from build123d import *

# Parameters (mm, degrees)
BOSS_EXTRUDE1_DEPTH = 4
SKETCH3_R           = 2
SKETCH3_R_2         = 2.25
CUT_EXTRUDE1_DEPTH  = 4


with BuildPart() as part:
    # Sketch2 → Boss-Extrude1 (new body)
    with BuildSketch(Plane.XY):
        with BuildLine():
            Line((94.375415976, -52.704406223), (94.375415976, -56.704406223))
            ThreePointArc((94.375415976, -56.704406223), (94.228969367, -57.057959614), (93.875415976, -57.204406223))
            Line((93.875415976, -57.204406223), (86.375415976, -57.204406223))
            ThreePointArc((86.375415976, -57.204406223), (86.021862586, -57.350852833), (85.875415976, -57.704406223))
            Line((85.875415976, -57.704406223), (85.875415976, -59.204406223))
            ThreePointArc((85.875415976, -59.204406223), (86.021862586, -59.557959614), (86.375415976, -59.704406223))
            Line((86.375415976, -59.704406223), (96.375415976, -59.704406223))
            ThreePointArc((96.375415976, -59.704406223), (96.728969367, -59.557959614), (96.875415976, -59.204406223))
            Line((96.875415976, -59.204406223), (96.875415976, -52.704406223))
            ThreePointArc((96.875415976, -52.704406223), (97.021862586, -52.350852833), (97.375415976, -52.204406223))
            Line((97.375415976, -52.204406223), (100.375415976, -52.204406223))
            ThreePointArc((100.375415976, -52.204406223), (106.756191002, -49.976139831), (110.36270914, -44.260154531))
            Line((110.36270914, -44.260154531), (122.04253828, 6.330743606))
            ThreePointArc((122.04253828, 6.330743606), (125.561092562, 11.907314631), (131.786238928, 14.081233063))
            Line((131.786238928, 14.081233063), (170.7844924, 14.081233063))
            ThreePointArc((170.7844924, 14.081233063), (180.903868338, 9.889650306), (185.095451094, -0.229725632))
            Line((185.095451094, -0.229725632), (185.095451094, -11.229725632))
            ThreePointArc((185.095451094, -11.229725632), (184.144121557, -18.570812299), (181.352982104, -25.42691337))
            ThreePointArc((181.352982104, -25.42691337), (169.65700257, -52.25234878), (163.771733482, -80.918766937))
            ThreePointArc((163.771733482, -80.918766937), (169.65700257, -109.585185095), (181.352982104, -136.410620505))
            ThreePointArc((181.352982104, -136.410620505), (184.144121557, -143.266721576), (185.095451094, -150.607808243))
            Line((185.095451094, -150.607808243), (185.095451094, -161.607808243))
            ThreePointArc((185.095451094, -161.607808243), (180.903868338, -171.727184181), (170.7844924, -175.918766937))
            Line((170.7844924, -175.918766937), (131.786238928, -175.918766937))
            ThreePointArc((131.786238928, -175.918766937), (125.561092562, -173.744848506), (122.04253828, -168.168277481))
            Line((122.04253828, -168.168277481), (110.36270914, -117.577379344))
            ThreePointArc((110.36270914, -117.577379344), (106.756191002, -111.861394044), (100.375415976, -109.633127651))
            Line((100.375415976, -109.633127651), (97.375415976, -109.633127651))
            ThreePointArc((97.375415976, -109.633127651), (96.668309195, -109.340234433), (96.375415976, -108.633127651))
            Line((96.375415976, -108.633127651), (96.375415976, -102.133127651))
            ThreePointArc((96.375415976, -102.133127651), (96.228969367, -101.779574261), (95.875415976, -101.633127651))
            Line((95.875415976, -101.633127651), (85.875415976, -101.633127651))
            ThreePointArc((85.875415976, -101.633127651), (85.521862586, -101.779574261), (85.375415976, -102.133127651))
            Line((85.375415976, -102.133127651), (85.375415976, -103.633127651))
            ThreePointArc((85.375415976, -103.633127651), (85.521862586, -103.986681042), (85.875415976, -104.133127651))
            Line((85.875415976, -104.133127651), (93.375415976, -104.133127651))
            ThreePointArc((93.375415976, -104.133127651), (93.728969367, -104.279574261), (93.875415976, -104.633127651))
            Line((93.875415976, -104.633127651), (93.875415976, -108.633127651))
            Line((93.875415976, -108.633127651), (93.875415976, -109.633127651))
            Line((93.875415976, -109.633127651), (82.315486211, -109.633127651))
            Line((82.315486211, -109.633127651), (79.315486211, -109.633127651))
            ThreePointArc((79.315486211, -109.633127651), (72.934711186, -111.861394044), (69.328193047, -117.577379344))
            Line((69.328193047, -117.577379344), (57.648363907, -168.168277481))
            ThreePointArc((57.648363907, -168.168277481), (54.129809626, -173.744848506), (47.904663259, -175.918766937))
            Line((47.904663259, -175.918766937), (8.906409788, -175.918766937))
            ThreePointArc((8.906409788, -175.918766937), (-1.21296615, -171.727184181), (-5.404548906, -161.607808243))
            Line((-5.404548906, -161.607808243), (-5.404548906, -150.607808243))
            ThreePointArc((-5.404548906, -150.607808243), (-4.453219369, -143.266721576), (-1.662079916, -136.410620505))
            ThreePointArc((-1.662079916, -136.410620505), (10.033899618, -109.585185095), (15.919168706, -80.918766937))
            ThreePointArc((15.919168706, -80.918766937), (10.033899618, -52.25234878), (-1.662079916, -25.42691337))
            ThreePointArc((-1.662079916, -25.42691337), (-4.453219369, -18.570812299), (-5.404548906, -11.229725632))
            Line((-5.404548906, -11.229725632), (-5.404548906, -0.229725632))
            ThreePointArc((-5.404548906, -0.229725632), (-1.21296615, 9.889650306), (8.906409788, 14.081233063))
            Line((8.906409788, 14.081233063), (47.904663259, 14.081233063))
            ThreePointArc((47.904663259, 14.081233063), (54.129809626, 11.907314631), (57.648363907, 6.330743606))
            Line((57.648363907, 6.330743606), (69.328193047, -44.260154531))
            ThreePointArc((69.328193047, -44.260154531), (72.934711186, -49.976139831), (79.315486211, -52.204406223))
            Line((79.315486211, -52.204406223), (82.315486211, -52.204406223))
            Line((82.315486211, -52.204406223), (93.875415976, -52.204406223))
            ThreePointArc((93.875415976, -52.204406223), (94.228969367, -52.350852833), (94.375415976, -52.704406223))
        make_face()
    extrude(amount=BOSS_EXTRUDE1_DEPTH)

    # Sketch3 → Cut-Extrude1 (cut)
    with BuildSketch(Plane.XY.offset(4)):
        with Locations((3.595451094, 3.081233063)):
            Circle(SKETCH3_R)
        with Locations((3.595451094, -166.918766937)):
            Circle(SKETCH3_R)
        with Locations((67.095451094, -60.918766937)):
            Circle(SKETCH3_R_2)
        with Locations((112.595451094, -60.918766937)):
            Circle(SKETCH3_R_2)
        with Locations((67.095451094, -100.918766947)):
            Circle(SKETCH3_R_2)
        with Locations((112.595451094, -100.918766947)):
            Circle(SKETCH3_R_2)
        with Locations((173.595451094, -166.918766937)):
            Circle(SKETCH3_R)
        with Locations((173.595451094, 3.081233063)):
            Circle(SKETCH3_R)
    extrude(amount=-CUT_EXTRUDE1_DEPTH, mode=Mode.SUBTRACT)


solid = part.part
Verification items for the finished model (mm, model axes). A direction names the side the tool comes from. Give positions to 0.01 mm unless a question says otherwise; leave off trailing zeros. Write each loop counter-clockwise with the first axis right and the second up, starting at its lowest first coordinate (ties: lowest second). Pieces come first, ordered by that corner, then holes. Notation, with made-up numbers: M -28.75,-3.5 L 7.25,-3.5 A22 ccw 7.25,18.5 Z; hole C -15.5,37.25 d5. An arc over 180 degrees is marked long. Use CSV: the item, a comma, the result in double quotes.
1) Go/stop test with flat-tipped pins: pin 1 Ø1.5 at (x, z) = (99, 1.5) entering from -Y; pin 2 Ø2.5 at (x, y) = (112.6, -60.92) entering from +Z; pin 3 Ø2 at (y, z) = (-104.5, 1.5) entering from -X; pin 4 Ø1.5 at (y, z) = (-91.5, 1.5) entering from -X. Record where each tip stops, or that it passes through.
Final values:
pin 1,"y = -109.63"
pin 2,"through"
pin 3,"x = 11.26"
pin 4,"x = 14.34"
2) Release check for a two-part mould opening along Y. For faces 1 (the face through (63.57, -142.52, 1.97)), 2 (the face through (125.49, 11.85, 1.97)), 3 (the face through (66.8, -98.69, 2.03)), 4 (the face through (9.9, -110, 2)) record: released by +Y, released by -Y, zero draft, split by the parting line, or undercut.
Final values:
face 1,"released by -Y"
face 2,"released by +Y"
face 3,"undercut"
face 4,"undercut"
3) Cross-section at D-D (z = 0.8). State how many separate pieces and enclosed holes the cut face has, plus the area to 3 significant figures.
Final values:
separate pieces,"1"
enclosed holes,"8"
area,"25,500 mm²"
4) Cross-section at C-C (x = 67). Enter the section's corners in (y, z), plus the area to 3 significant figures.
Final values:
outline,"M -127.66,0 L -103.17,0 L -103.17,4 L -127.66,4 Z; M -98.67,0 L -63.17,0 L -63.17,4 L -98.67,4 Z; M -58.67,0 L -34.18,0 L -34.18,4 L -58.67,4 Z"
area,"338 mm²"
5) Material ranges on line 1 along X through (y, z) = (-26, 3.35); line 2 along X through (y, z) = (-50.5, 2.2); line 3 along Y through (x, z) = (82.5, 3.7), recorded low to high.
Final values:
line 1,"-1.34 to 65.11, 114.58 to 181.03"
line 2,"9.47 to 73.66, 106.04 to 170.22"
line 3,"-109.63 to -52.2"
6) Access from +Z, -Z, +X, -X, +Y, -Y to the whole of each face (thin tool, end or side, straight path). Record for faces 5 (the face through (180.79, 10, 1.97)), 6 (the face through (10.157, -52.644, 1.972)), 7 (the face through (106.83, -111.92, 1.97)), 8 (the face through (116.12, -19.32, 1.97)), 9 (the face through (169.78, -51.86, 1.97)).
Final values:
face 5,"+Z, -Z, +X, +Y"
face 6,"+Z, -Z, -X"
face 7,"+Z, -Z, -Y"
face 8,"+Z, -Z, +Y"
face 9,"+Z, -Z, +X"
7) Cross-section at A-A (x = 168.5). Enter the section's corners in (y, z), plus the area to 3 significant figures.
Final values:
outline,"M -175.92,0 L -105.74,0 L -105.74,4 L -175.92,4 Z; M -56.09,0 L 14.08,0 L 14.08,4 L -56.09,4 Z"
area,"561 mm²"
8) Cross-section at B-B (y = -129). Enter the section's corners in (x, z), plus the area to 3 significant figures.
Final values:
outline,"M 2.25,0 L 66.69,0 L 66.69,4 L 2.25,4 Z; M 113,0 L 177.44,0 L 177.44,4 L 113,4 Z"
area,"516 mm²"
